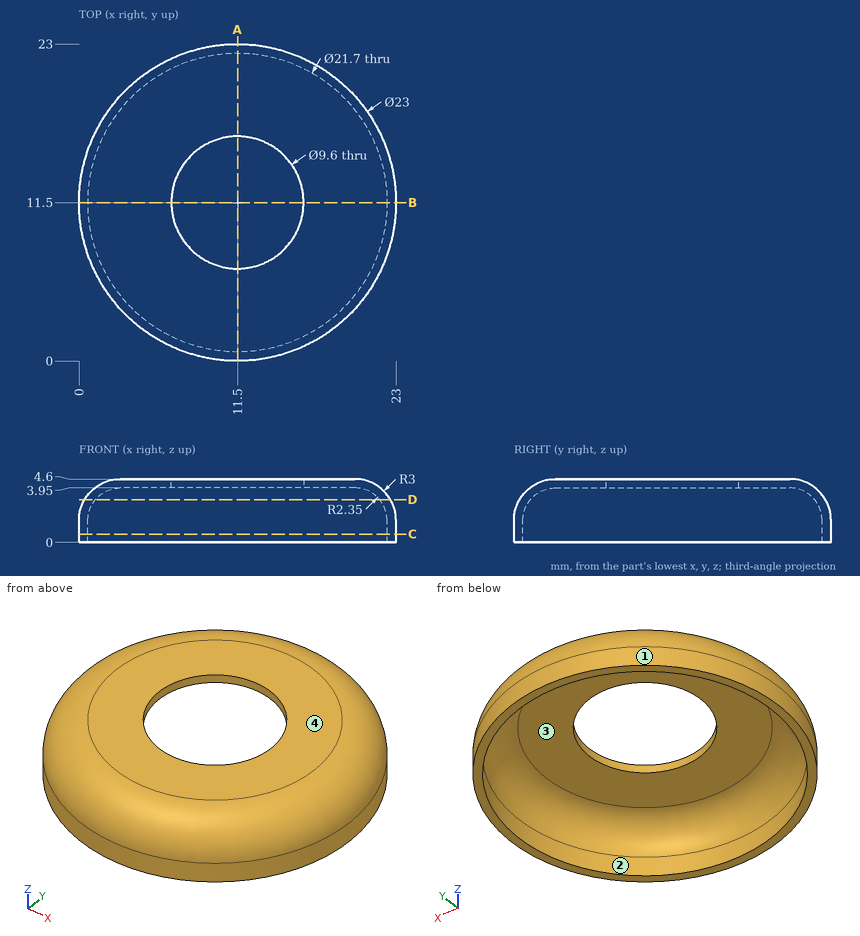
For this review, use the dimensioned drawing (mm, ordinates from the lowest corner) and the shaded views. Round coordinates to 2 decimals unless told otherwise and drop trailing zeros. Write each loop counter-clockwise with the first axis right and the second up, starting at its lowest first coordinate (ties: lowest second). Pieces come first, ordered by that corner, then holes. Notation, with made-up numbers: (-38, 47.25) -> (-13, 47.25) arc R21 cw to (-13, 72.25) -> close; hole circle Ø7 at (46.5, 71.25). An arc over 180 degrees is marked (long way). Use one line per item in the form item = value.
Q1. Consider section A-A (x = 11.5). State the section outline as (y, z) points.
Resolved:
outline = (0, 0) -> (0.65, 0) -> (0.65, 1.6) arc R2.35 cw to (3, 3.95) -> (6.7, 3.95) -> (6.7, 4.6) -> (3, 4.6) arc R3 ccw to (0, 1.6) -> close; (16.3, 3.95) -> (20, 3.95) arc R2.35 cw to (22.35, 1.6) -> (22.35, 0) -> (23, 0) -> (23, 1.6) arc R3 ccw to (20, 4.6) -> (16.3, 4.6) -> close
Q2. Consider section C-C (z = 0.6). State the section outline as (x, y) points.
Resolved:
outline = circle Ø23 at (11.5, 11.5); hole circle Ø21.7 at (11.5, 11.5)
Q3. The part is to be moulded in two halves that separate along X. For the marked faces 1, 2, 3 and 4, say which applies: released by +X, released by -X, zero draft, split by the parting line, or undercut.
Resolved:
face_1 = split by the parting line
face_2 = undercut
face_3 = undercut
face_4 = zero draft
Q4. Consider section D-D (z = 3.1). State the section outline as (x, y) points, then the cut area to 3 significant figures.
Resolved:
outline = circle Ø22.2 at (11.5, 11.5); hole circle Ø20.62 at (11.5, 11.5)
area = 53.1 mm²
Q5. To check wall thickness, follow probe 1 along X at (y, z) = (11.5, 1.35); probe 2 along Y at (x, z) = (11.5, 4.2); probe 3 along X at (y, z) = (10, 3.7). State the ranges of each line that lie inside material, in increasing order. Write a range as from..to.
Resolved:
probe_1 = 0..0.65, 22.35..23
probe_2 = 1.5..6.7, 16.3..21.5
probe_3 = 0.96..2.06, 20.94..22.04
Q6. Clearance check with flat-ended pins moving along their axes: pin 1 Ø1 at (y, z) = (10, 1) entering from -X; pin 2 Ø8.5 at (x, y) = (8.5, 7.5) entering from -Z; pin 3 Ø4 at (x, y) = (19.5, 13) entering from -Z. State where each tip first meets the part, or that it passes through.
Resolved:
pin_1 = 0.04
pin_2 = 3.83
pin_3 = 3.28
